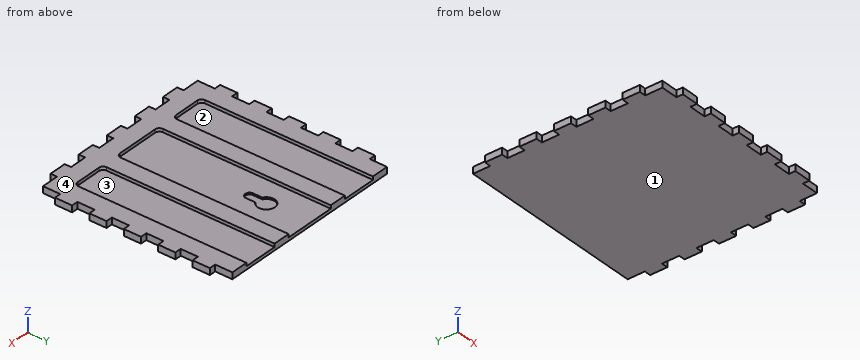
from build123d import *

# Parameters (mm, degrees)
SKETCH2_W               = 279.4
SKETCH2_H               = 279.4
BOSS_EXTRUDE1_DEPTH     = 9.525
SKETCH4_W               = 9.525
SKETCH4_H               = 25.4
BOSS_EXTRUDE3_DEPTH     = 9.525
LPATTERN2_COUNT         = 5
LPATTERN2_PITCH         = 50.8
MIRROR2_COPY_1_SKETCH_W = 9.525
MIRROR2_COPY_1_SKETCH_H = 25.4
MIRROR2_COPY_1_DEPTH    = 9.525
MIRROR2_COPY_2_SKETCH_W = 9.525
MIRROR2_COPY_2_SKETCH_H = 25.4
MIRROR2_COPY_2_DEPTH    = 9.525
MIRROR2_COPY_3_SKETCH_W = 9.525
MIRROR2_COPY_3_SKETCH_H = 25.4
MIRROR2_COPY_3_DEPTH    = 9.525
MIRROR2_COPY_4_SKETCH_W = 9.525
MIRROR2_COPY_4_SKETCH_H = 25.4
MIRROR2_COPY_4_DEPTH    = 9.525
SKETCH5_W               = 25.4
SKETCH5_H               = 9.525
BOSS_EXTRUDE4_DEPTH     = 9.525
LPATTERN3_COUNT         = 5
LPATTERN3_PITCH         = 50.8
SKETCH6_W               = 76.2
SKETCH6_H               = 254
SKETCH6_W_2             = 50.8
CUT_EXTRUDE1_DEPTH      = 4.7625
FILLET1_R               = 6.35
CUT_EXTRUDE2_DEPTH      = 2.54


with BuildPart() as part:
    # Sketch2 → Boss-Extrude1 (new body)
    with BuildSketch(Plane.XY):
        Rectangle(SKETCH2_W, SKETCH2_H)
    extrude(amount=BOSS_EXTRUDE1_DEPTH)

    # Sketch4 → Boss-Extrude3 (add)
    with BuildSketch(Plane(origin=(139.7, 0, 0), x_dir=(0, 0, -1), z_dir=(1, 0, 0))):
        with Locations((-4.7625, -101.6)):
            Rectangle(SKETCH4_W, SKETCH4_H)
    boss_extrude3 = extrude(amount=BOSS_EXTRUDE3_DEPTH)

    # LPattern2: Boss-Extrude3 ×5
    with Locations(*[(0, i * LPATTERN2_PITCH, 0) for i in range(1, LPATTERN2_COUNT)]):
        add(boss_extrude3)

    # Mirror2: Boss-Extrude3 across plane
    add(boss_extrude3.mirror(Plane(origin=(0, 0, 0), x_dir=(0, 0, 1), z_dir=(1, 0, 0))))

    # Mirror2 copy 1 sketch → Mirror2 copy 1 (add)
    with BuildSketch(Plane(origin=(-139.7, 50.8, 0), x_dir=(0, 0, -1), z_dir=(-1, 0, 0))):
        with Locations((-4.7625, 101.6)):
            Rectangle(MIRROR2_COPY_1_SKETCH_W, MIRROR2_COPY_1_SKETCH_H)
    extrude(amount=MIRROR2_COPY_1_DEPTH)

    # Mirror2 copy 2 sketch → Mirror2 copy 2 (add)
    with BuildSketch(Plane(origin=(-139.7, 101.6, 0), x_dir=(0, 0, -1), z_dir=(-1, 0, 0))):
        with Locations((-4.7625, 101.6)):
            Rectangle(MIRROR2_COPY_2_SKETCH_W, MIRROR2_COPY_2_SKETCH_H)
    extrude(amount=MIRROR2_COPY_2_DEPTH)

    # Mirror2 copy 3 sketch → Mirror2 copy 3 (add)
    with BuildSketch(Plane(origin=(-139.7, 152.4, 0), x_dir=(0, 0, -1), z_dir=(-1, 0, 0))):
        with Locations((-4.7625, 101.6)):
            Rectangle(MIRROR2_COPY_3_SKETCH_W, MIRROR2_COPY_3_SKETCH_H)
    extrude(amount=MIRROR2_COPY_3_DEPTH)

    # Mirror2 copy 4 sketch → Mirror2 copy 4 (add)
    with BuildSketch(Plane(origin=(-139.7, 203.2, 0), x_dir=(0, 0, -1), z_dir=(-1, 0, 0))):
        with Locations((-4.7625, 101.6)):
            Rectangle(MIRROR2_COPY_4_SKETCH_W, MIRROR2_COPY_4_SKETCH_H)
    extrude(amount=MIRROR2_COPY_4_DEPTH)

    # Sketch5 → Boss-Extrude4 (add)
    with BuildSketch(Plane.XZ.offset(139.7)):
        with Locations((-101.6, 4.7625)):
            Rectangle(SKETCH5_W, SKETCH5_H)
    boss_extrude4 = extrude(amount=BOSS_EXTRUDE4_DEPTH)

    # LPattern3: Boss-Extrude4 ×5
    with Locations(*[(i * LPATTERN3_PITCH, 0, 0) for i in range(1, LPATTERN3_COUNT)]):
        add(boss_extrude4)

    # Sketch6 → Cut-Extrude1 (cut)
    with BuildSketch(Plane.XY.offset(9.525)):
        with Locations((0, 12.7)):
            Rectangle(SKETCH6_W, SKETCH6_H)
        with Locations((-88.9, 12.7)):
            Rectangle(SKETCH6_W_2, SKETCH6_H)
        with Locations((88.9, 12.7)):
            Rectangle(SKETCH6_W_2, SKETCH6_H)
    extrude(amount=-CUT_EXTRUDE1_DEPTH, mode=Mode.SUBTRACT)

    # Fillet1
    fillet1_edges = [part.edges().sort_by_distance(p)[0] for p in [
        (63.5, -114.3, 7.14375),
        (114.3, -114.3, 7.14375),
        (-114.3, -114.3, 7.14375),
        (-63.5, -114.3, 7.14375),
        (-38.1, -114.3, 7.14375),
        (38.1, -114.3, 7.14375),
    ]]
    fillet(fillet1_edges, radius=FILLET1_R)

    # Sketch7 → Cut-Extrude2 (cut)
    with BuildSketch(Plane.XY.offset(4.7625)):
        with BuildLine():
            Line((6.35, 64.711297153), (6.35, 51.001361114))
            ThreePointArc((6.35, 51.001361114), (0, 44.651361114), (-6.35, 51.001361114))
            Line((-6.35, 51.001361114), (-6.35, 64.711297153))
            ThreePointArc((-6.35, 64.711297153), (0, 88.409819781), (6.35, 64.711297153))
        make_face()
    extrude(amount=-CUT_EXTRUDE2_DEPTH, mode=Mode.SUBTRACT)


solid = part.part
Model file for the job. Use its own axes, mm. Face numbers are marked on the shaded views. A direction names the side the tool comes from. Give positions to 0.01 mm unless a question says otherwise; leave off trailing zeros. Loops run counter-clockwise (first coordinate to the right, second up) from the corner with the lowest first, then second, coordinate; pieces in that order, holes last. Notation, with made-up numbers: (35, -13.5) -> (80, -13.5) arc R33 ccw to (80, 17.5) -> close; hole circle Ø6 at (23.25, 20). An arc over 180 degrees is marked (long way). Use a Markdown table: item, result. Add a question column.
(1) Slice it at D-D on x = 100.5. List the corners of the cut face in (y, z) (1 decimal), and give its area (3 significant figures).
(2) Wall check: line 1 along X through (y, z) = (-31, 8.75); line 2 along X through (y, z) = (-2.5, 9) (3 decimals); line 3 along Y through (x, z) = (0, 3.1) (3 decimals). Give the ranges that are in metal, low to high.
(3) Slice it at C-C on x = -74. List the corners of the cut face in (y, z) (1 decimal), and give its area (3 significant figures).
(4) Slice it at A-A on x = 0. List the corners of the cut face in (y, z) (1 decimal).
(5) Drop flat-ended pins along their axis: pin 1 Ø5 at (x, z) = (146, 4) entering from -Y; pin 2 Ø5 at (y, z) = (-75.5, 3.5) entering from -X; pin 3 Ø4 at (x, z) = (76.5, 2.5) entering from -Y. Give the stop position or say it passes through.
(6) Tool access for the marked faces 3 and 4: list every direction of +Z, -Z, +X, -X, +Y, -Y with a clear straight run to the whole face (end or side of a thin tool).
(7) Mould opens along X. For the marked faces 1 and 2 say: +X half, -X half, draft (parallel to the pull), parting line (faces both ways), or undercut.
(8) Slice it at B-B on y = -23.5. List the corners of the cut face in (x, z) (1 decimal).
Filled sheet:
| question | item | result |
|---|---|---|
| 1 | outline | (-149.2, 0) -> (139.7, 0) -> (139.7, 4.8) -> (-114.3, 4.8) -> (-114.3, 9.5) -> (-149.2, 9.5) -> close |
| 1 | area | 1,540 mm2 |
| 2 | line 1 | -139.7 to -114.3, -63.5 to -38.1, 38.1 to 63.5, 114.3 to 139.7 |
| 2 | line 2 | -149.225 to -114.3, -63.5 to -38.1, 38.1 to 63.5, 114.3 to 149.225 |
| 2 | line 3 | -149.225 to 44.651, 88.41 to 139.7 |
| 3 | outline | (-139.7, 0) -> (139.7, 0) -> (139.7, 4.8) -> (-114.3, 4.8) -> (-114.3, 9.5) -> (-139.7, 9.5) -> close |
| 3 | area | 1,450 mm2 |
| 4 | outline | (-149.2, 0) -> (139.7, 0) -> (139.7, 4.8) -> (88.4, 4.8) -> (88.4, 2.2) -> (44.7, 2.2) -> (44.7, 4.8) -> (-114.3, 4.8) -> (-114.3, 9.5) -> (-149.2, 9.5) -> close |
| 5 | pin 1 | y = -114.3 |
| 5 | pin 2 | x = -139.7 |
| 5 | pin 3 | y = -139.7 |
| 6 | face 3 | +Z, +Y |
| 6 | face 4 | +Z, +X, -X, +Y, -Y |
| 7 | face 1 | draft |
| 7 | face 2 | undercut |
| 8 | outline | (-139.7, 0) -> (139.7, 0) -> (139.7, 9.5) -> (114.3, 9.5) -> (114.3, 4.8) -> (63.5, 4.8) -> (63.5, 9.5) -> (38.1, 9.5) -> (38.1, 4.8) -> (-38.1, 4.8) -> (-38.1, 9.5) -> (-63.5, 9.5) -> (-63.5, 4.8) -> (-114.3, 4.8) -> (-114.3, 9.5) -> (-139.7, 9.5) -> close |
